from build123d import *

# Parameters (mm, degrees)
SKETCH3_OUTSIDE_W  = 36.488
SKETCH3_OUTSIDE_H  = 36.488
CUT_EXTRUDE1_DEPTH = 46.03250001
CHAMFER1_SIZE      = 0.508
FILLET1_R          = 0.635


with BuildPart() as part:
    # Sketch2 → Revolve1 (revolve)
    with BuildSketch(Plane(origin=(0, 0, 0), x_dir=(0, 0, -1), z_dir=(1, 0, 0)), mode=Mode.PRIVATE) as revolve1_sk:
        Polygon((0, 3.175), (0, 6.35), (7.9502, 6.35), (7.9502, 7.62), (53.98270001, 7.62), (53.98270001, 9.525), (60.33270001, 9.525), (60.33270001, 8.5), (72.33270001, 8.5), (72.33270001, 0), (6.858, 0), (6.858, 3.175), align=None)
    revolve(revolve1_sk.sketch.rotate(Axis((0, 0, 0), (0, 0, 1)), 90), axis=Axis((0, 0, 0), (0, 0, 1)))

    # Sketch3 outside → Cut-Extrude1 (cut)
    with BuildSketch(Plane.XY.offset(-7.9502)):
        Rectangle(SKETCH3_OUTSIDE_W, SKETCH3_OUTSIDE_H)
        Polygon((3.696970073, 6.40334), (-3.696970073, 6.40334), (-7.393940145, 0), (-3.696970073, -6.40334), (3.696970073, -6.40334), (7.393940145, 0), align=None, mode=Mode.SUBTRACT)
    extrude(amount=-CUT_EXTRUDE1_DEPTH, mode=Mode.SUBTRACT)

    # Chamfer1
    chamfer1_edges = [part.edges().sort_by_distance(p)[0] for p in [
        (8.5, 0, -72.33270001),
        (6.35, 0, 0),
    ]]
    chamfer(chamfer1_edges, length=CHAMFER1_SIZE)

    # Fillet1
    fillet1_edges = [part.edges().sort_by_distance(p)[0] for p in [
        (3.696970073, 6.40334, -30.966450005),
        (-3.696970073, 6.40334, -30.966450005),
        (-7.393940145, 0, -30.966450005),
        (-3.696970073, -6.40334, -30.966450005),
        (3.696970073, -6.40334, -30.966450005),
        (7.393940145, 0, -30.966450005),
    ]]
    fillet(fillet1_edges, radius=FILLET1_R)


solid = part.part
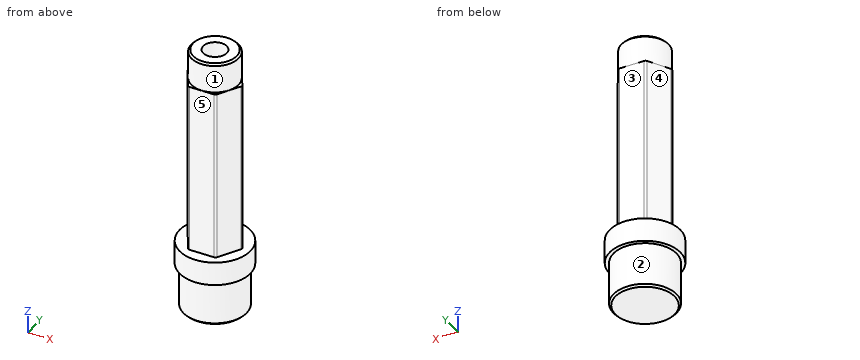
Design review of the part built by this model. Coordinates are the model's own, in mm. Face numbers are marked on the shaded views. A direction names the side the tool comes from. Coordinates: 2 decimals unless noted, no trailing zeros. Loops run counter-clockwise (first coordinate to the right, second up) from the corner with the lowest first, then second, coordinate; pieces in that order, holes last. Notation, with made-up numbers: (28, -25) - (68, -25) arc R21 cw to (68, 7) - close; hole circle Ø7 at (67, 55.25). An arc over 180 degrees is marked (long way). Use CSV: the item, a comma, the result in double quotes. Start each with the question number.
1. Add section B-B on x = 0. Give the boundary of the cut face in (y, z) (3 decimals).
2. For the marked faces 1, 2, 3, 4 and 5, list the 3-axis set-ups (+Z, -Z, +X, -X, +Y, -Y) from which the entire face can be reached by the end or side of a thin tool; tool diameter is ignored.
3. Add section C-C on z = -32. Give the boundary of the cut face in (x, y) (1 decimal), plus the area to 3 significant figures.
4. Clearance check with flat-ended pins moving along their axes: pin 1 (1.5 mm diameter, centred on x = -0.5, z = -13, fed in from +Y); pin 2 (2 mm diameter, centred on y = 2, z = -37.5, fed in from +X); pin 3 (5.5 mm diameter, centred on x = -1, z = -21, fed in from -Y). State where each tip first meets the part, or that it passes through.
5. To check wall thickness, follow probe 1 along Y at (x, z) = (0, -3.5) (3 decimals); probe 2 along Z at (x, y) = (0, -7.75); probe 3 along Y at (x, z) = (-2.75, -9). State the ranges of each line that lie inside material, in increasing order.
6. Add section A-A on z = -6. Give the boundary of the cut face in (x, y) (3 decimals).
7. Add section D-D on z = -66. Give the boundary of the cut face in (x, y).
Resolved:
1,outline,"(-9.525, -60.333) - (-8.5, -60.333) - (-8.5, -71.825) - (-7.992, -72.333) - (7.992, -72.333) - (8.5, -71.825) - (8.5, -60.333) - (9.525, -60.333) - (9.525, -53.983) - (6.403, -53.983) - (6.403, -7.95) - (6.35, -7.95) - (6.35, -0.508) - (5.842, 0) - (3.175, 0) - (3.175, -6.858) - (-3.175, -6.858) - (-3.175, 0) - (-5.842, 0) - (-6.35, -0.508) - (-6.35, -7.95) - (-6.403, -7.95) - (-6.403, -53.983) - (-9.525, -53.983) - close"
2,face 1,"+Z"
2,face 2,"-Z"
2,face 3,"+Z, +X, -X, +Y"
2,face 4,"+Z, -X, +Y"
2,face 5,"+Z, +X, -X, -Y"
3,outline,"(-7.2, -0.3) - (-3.9, -6.1) arc R0.6 ccw to (-3.3, -6.4) - (3.3, -6.4) arc R0.6 ccw to (3.9, -6.1) - (7.2, -0.3) arc R0.6 ccw to (7.2, 0.3) - (3.9, 6.1) arc R0.6 ccw to (3.3, 6.4) - (-3.3, 6.4) arc R0.6 ccw to (-3.9, 6.1) - (-7.2, 0.3) arc R0.6 ccw to start"
3,area,"142 mm2"
4,pin 1,"y = 6.4"
4,pin 2,"x = 6.82"
4,pin 3,"y = -6.4"
5,probe 1,"-6.35 to -3.175, 3.175 to 6.35"
5,probe 2,"-72.33 to -53.98"
5,probe 3,"-6.4 to 6.4"
6,outline,"circle Ø12.7 at (0, 0); hole circle Ø6.35 at (0, 0)"
7,outline,"circle Ø17 at (0, 0)"
